Could you check a few things on this model? Use its own coordinates, in mm. A direction names the side the tool comes from. Round coordinates to 2 decimals unless told otherwise and drop trailing zeros. Write each loop counter-clockwise with the first axis right and the second up, starting at its lowest first coordinate (ties: lowest second). Pieces come first, ordered by that corner, then holes. Notation, with made-up numbers: M 53,-11 L 74,-11 A23 ccw 74,3 Z; hole C -32.5,-4.75 d11. An arc over 180 degrees is marked long. One line per item, written item: value. Start each with the question number.
(1) I want a section at B-B on y = -3.1. Please give me the cut outline in (x, z), and give its area (3 significant figures).
(2) I want a section at D-D on z = 5.75. Please give me the cut outline in (x, y), and give its area (3 significant figures).
(3) I want a section at A-A on x = 1. Please give me the cut outline in (y, z), and give its area (3 significant figures).
(4) Which directions (+Z, -Z, +X, -X, +Y, -Y) give clear straight access to the entire face, cutting with the end or side of a thin tool? Please do faces 4 (the face through (2.07, -0.24, 13.77)), 5 (the face through (5.236, -4.759, 15.659)), 6 (the face through (6, -5, 7)), 7 (the face through (5.008, -2, 16)), 8 (the face through (0, -2, 12)).
(5) I'm going to push flat-ended pins straight in: pin 1 Ø1.2 at (y, z) = (-2, 16) entering from -X; pin 2 Ø3 at (x, y) = (2, -1) entering from -Z. Where does each tip first touch, or does it pass through?
(6) I want a section at C-C on z = 15.75. Please give me the cut outline in (x, y).
(7) If I drill on L1, parallel to Z at x = 2.25, y = -3.15; L2, parallel to X at y = -3.2, z = 4.75, over which ranges is the centre line in solid material (lowest first)?
(8) Thinking about a two-plate mould opening in Z: for faces 1 (the face through (4, -2, 0)), 2 (the face through (2.07, -4.76, 13.77)), 3 (the face through (8, -2, 8)), which applies, released by +Z, released by -Z, zero draft, split by the parting line, or undercut?
```python
from build123d import *

# Parameters (mm, degrees)
F1_DEPTH = 5
F2_R     = 0.8


with BuildPart() as f1:
    # F0 (on Front) → F1 (new body)
    with BuildSketch(Plane.XZ):
        Polygon((0, 3), (0, 0), (8, 0), (8, 18), (0, 18), (0, 16.25), (5.0083114872, 16.25), (5.0083114872, 14), (0, 14), (0, 11), (5, 11), (5, 3), align=None)
    extrude(amount=F1_DEPTH)

    # F2
    f2_edges = [f1.edges().sort_by_distance(p)[0] for p in [
        (0, -2.5, 18),
        (0, -2.5, 16.25),
        (2.504156, -5, 14),
        (5.008311, -5, 15.125),
        (5.008311, 0, 15.125),
        (2.504156, -5, 16.25),
        (2.504156, 0, 14),
        (2.504156, 0, 16.25),
        (4, 0, 18),
        (4, -5, 18),
        (8, -2.5, 18),
        (5.008311, -2.5, 14),
        (0, -2.5, 14),
    ]]
    fillet(f2_edges, radius=F2_R)


solid = f1.part
```
Found:
1. outline: M 0,0 L 8,0 L 8,17.2 A0.8 ccw 7.2,18 L 0.8,18 A0.8 ccw 0,17.2 L 0,17.05 A0.8 ccw 0.8,16.25 L 5.01,16.25 L 5.01,14.8 A0.8 cw 4.21,14 L 0.8,14 A0.8 ccw 0,13.2 L 0,11 L 5,11 L 5,3 L 0,3 Z
1. area: 92.3 mm²
2. outline: M 5,-5 L 8,-5 L 8,0 L 5,0 Z
2. area: 15.0 mm²
3. outline: M -5,0 L 0,0 L 0,3 L -5,3 Z; M -5,11 L 0,11 L 0,13.2 A0.8 ccw -0.8,14 L -4.2,14 A0.8 ccw -5,13.2 Z; M -5,17.05 A0.8 ccw -4.2,16.25 L -0.8,16.25 A0.8 ccw 0,17.05 L 0,17.2 A0.8 ccw -0.8,18 L -4.2,18 A0.8 ccw -5,17.2 Z
3. area: 37.9 mm²
4. face 4: -X, +Y
4. face 5: -X, -Y
4. face 6: +Z, -Z, +X, -X, -Y
4. face 7: -X, +Y, -Y
4. face 8: +Z, -Z, -X, +Y, -Y
5. pin 1: stops at x = 0.14
5. pin 2: stops at z = 0
6. outline: M 5.01,-4.2 A0.8 ccw 5.81,-5 L 8,-5 L 8,0 L 5.81,0 A0.8 ccw 5.01,-0.8 Z
7. L1: z = 0 to 3, 11 to 14, 16.25 to 18
7. L2: x = 5 to 8
8. face 1: released by -Z
8. face 2: undercut
8. face 3: zero draft
